Input: part model. Units: mm. Frame: model coordinates. A direction names the side the tool comes from. Give positions to 0.01 mm unless a question says otherwise; leave off trailing zeros. Loops run counter-clockwise (first coordinate to the right, second up) from the corner with the lowest first, then second, coordinate; pieces in that order, holes last.
from build123d import *

# Parameters (mm, degrees)
SKETCH_1_W      = 2.54
SKETCH_1_H      = 2.54
EXTRUDE_1_DEPTH = 2.54
SKETCH_2_W      = 0.67
SKETCH_2_H      = 0.67
FILLET_1_R      = 0.5


with BuildPart() as part:
    # 草图1 → 拉伸1 (new body)
    with BuildSketch(Plane.XY):
        with Locations((0, -1.289090726)):
            Rectangle(SKETCH_1_W, SKETCH_1_H)
    extrude(amount=EXTRUDE_1_DEPTH)

    # 扫描1: sweep along a path in 草图3
    with BuildLine(Plane(origin=(0, 0, 0), x_dir=(0, 0, -1), z_dir=(1, 0, 0))) as sweep_1_path:
        Line((-7.62, -1.299090726), (0.5, -1.299090726))
        Line((0.5, -1.299090726), (12.787280664, -9.902737271))
    # 草图2 → 扫描1 (sweep)
    with BuildSketch(Plane(origin=(0, 0, 7.62), x_dir=(-1, 0, 0), z_dir=(0, 0, -1))):
        with Locations((0, -1.289090726)):
            Rectangle(SKETCH_2_W, SKETCH_2_H)
    sweep(path=sweep_1_path.line, transition=Transition.RIGHT)

    # 圆角1
    fillet_1_edges = [part.edges().sort_by_distance(p)[0] for p in [
        (-1.27, -0.019090726, 1.27),
        (1.27, -0.019090726, 1.27),
        (1.27, -2.559090726, 1.27),
        (-1.27, -2.559090726, 1.27),
    ]]
    fillet(fillet_1_edges, radius=FILLET_1_R)


solid = part.part
(1) Cut plane B-B (z = 6). Return the cut outline in (x, y) (3 decimals).
Values follow:
outline: (-0.335, -1.624) - (0.335, -1.624) - (0.335, -0.954) - (-0.335, -0.954) - close
(2) Cut plane C-C (y = -8.5). Return the cut outline in (x, z) (3 decimals), and give its area (3 significant figures).
Values follow:
outline: (-0.335, -11.385) - (0.335, -11.385) - (0.335, -10.217) - (-0.335, -10.217) - close
area: 0.783 mm2
(3) Pin query (flat end, axial travel): pin 1 Ø3 at (y, z) = (-6, -5.5) entering from +X (3 decimals); pin 2 Ø1.3 at (x, y) = (-0.5, -2) entering from -Z; pin 3 Ø1.5 at (x, y) = (0, -6.5) entering from -Z. Return the tip coordinate at first contact, or that it passes through.
Values follow:
pin 1: stops at x = 0.335
pin 2: stops at z = -3
pin 3: stops at z = -9.6
(4) Reachability of faces 1 (the flat face through (1, -1, 0)), 2 (the flat face through (0.335, -5, -6)), 3 (the flat face through (0, -2.559, 1)), 4 (the flat face through (-0.335, -5, -6)), 5 (the flat face through (1.27, -1, 1)) from +Z, -Z, +X, -X, +Y, -Y: full face, straight path, thin tool, end or side. Return the list, or none.
Values follow:
face 1: none
face 2: -Z, +X, +Y, -Y
face 3: +Z, +X, -X, -Y
face 4: -Z, -X, +Y, -Y
face 5: +Z, -Z, +X, +Y, -Y
(5) Cut plane A-A (x = 0.1). Return the cut outline in (y, z).
Values follow:
outline: (-10.17, -12.6) - (-9.62, -12.99) - (-0.95, -0.61) - (-0.95, 0) - (-0.02, 0) - (-0.02, 2.54) - (-0.95, 2.54) - (-0.95, 7.62) - (-1.62, 7.62) - (-1.62, 2.54) - (-2.56, 2.54) - (-2.56, 0) - (-1.62, 0) - (-1.62, -0.4) - close
(6) Ray query, probe 1 along Y at (x, z) = (0.75, 1.25); probe 2 along Z at (x, y) = (0.2, -0.5); probe 3 along Z at (x, y) = (-0.3, -2). Return the intervals inside material, ascending.
Values follow:
probe 1: y = -2.56 to -0.02
probe 2: z = 0 to 2.54
probe 3: z = -2.1 to -0.93, 0 to 2.54
